The model under review builds one solid part; all positions refer to its coordinate system, in mm. A direction names the side the tool comes from. Coordinates: 2 decimals unless noted, no trailing zeros. Write each loop counter-clockwise with the first axis right and the second up, starting at its lowest first coordinate (ties: lowest second). Pieces come first, ordered by that corner, then holes. Notation, with made-up numbers: (79.5, 34) - (86.5, 34) arc R12 ccw to (86.5, 42) - close; hole circle Ø7 at (82.25, 85.25). An arc over 180 degrees is marked (long way). Return JSON: item names as keys, results as strings. Group by question number.
(1) For pin 1 Ø12 at (y, z) = (-9, 12) entering from +X; pin 2 Ø3 at (x, z) = (-2.5, 12) entering from -Y; pin 3 Ø1.5 at (y, z) = (-12.5, 15.5) entering from +X, all flat-tipped, find the tip position at first contact; note any pin that passes through.
(2) To check wall thickness, follow L1, parallel to Z at x = -10.5, y = -15; L2, parallel to X at y = 15.25, z = 9.5; L3, parallel to Y at x = 15.25, z = -1.5. State the ranges of each line that lie inside material, in increasing order. Write a range as from..to.
(3) We need section B-B on x = 15.25. Give the number of separate pieces and of enclosed holes in the cut face, then the cut area to 3 significant figures.
(4) We need section C-C on y = -7.5. State the section outline as (x, z) points.
(5) Draft analysis for pull direction Y (two halves, no side actions). For faces 1 (the face through (-18, 0, 10)), 2 (the face through (0, 0, 2)), 3 (the face through (0, 18, 10)), state which applies: released by +Y, released by -Y, zero draft, split by the parting line, or undercut.
(6) We need section A-A on z = 4.25. State the section outline as (x, y) points, then the cut area to 3 significant figures.
(7) We need section D-D on x = -6.5. State the section outline as (y, z) points, then the cut area to 3 significant figures.
(8) Tool access review of faces 4 (the face through (-17.551, 17.015, -2.465)), 5 (the face through (17.5, 17.5, 0)), 6 (the face through (-17.551, -17.015, 5.451)): name each direction out of +Z, -Z, +X, -X, +Y, -Y from which nothing blocks a thin tool from reaching the whole face with its end or side.
```python
from build123d import *

# Parameters (mm, degrees)
SKETCH_W      = 36
SKETCH_H      = 36
SKETCH_R      = 1.5
PAD_DEPTH     = 2
SKETCH001_R   = 2.9
SKETCH001_R_2 = 1.5
PAD001_DEPTH  = 7
SKETCH002_W   = 36
SKETCH002_H   = 36
SKETCH002_R   = 1.5
PAD002_DEPTH  = 2
SKETCH003_R   = 2.9
SKETCH003_R_2 = 1.5
PAD003_DEPTH  = 5
SKETCH004_W   = 18
SKETCH004_H   = 36
PAD004_DEPTH  = 2
SKETCH005_R   = 2.9
SKETCH005_R_2 = 1.5
PAD005_DEPTH  = 5


with BuildPart() as part:
    # Sketch → Pad (new body)
    with BuildSketch(Plane.XY):
        Rectangle(SKETCH_W, SKETCH_H)
        with Locations((-15.25, -15.25)):
            Circle(SKETCH_R, mode=Mode.SUBTRACT)
        with Locations((15.25, -15.25)):
            Circle(SKETCH_R, mode=Mode.SUBTRACT)
        with Locations((-15.25, 15.25)):
            Circle(SKETCH_R, mode=Mode.SUBTRACT)
        with Locations((15.25, 15.25)):
            Circle(SKETCH_R, mode=Mode.SUBTRACT)
    extrude(amount=PAD_DEPTH)

    # Sketch001 (on Face10 of Pad) → Pad001 (join)
    with BuildSketch(Plane.XY.offset(2)):
        with Locations((-15.25, 15.25)):
            Circle(SKETCH001_R)
        with Locations((-15.25, 15.25)):
            Circle(SKETCH001_R_2, mode=Mode.SUBTRACT)
        with Locations((-15.25, -15.25)):
            Circle(SKETCH001_R)
        with Locations((-15.25, -15.25)):
            Circle(SKETCH001_R_2, mode=Mode.SUBTRACT)
        with Locations((15.25, -15.25)):
            Circle(SKETCH001_R)
        with Locations((15.25, -15.25)):
            Circle(SKETCH001_R_2, mode=Mode.SUBTRACT)
        with Locations((15.25, 15.25)):
            Circle(SKETCH001_R)
        with Locations((15.25, 15.25)):
            Circle(SKETCH001_R_2, mode=Mode.SUBTRACT)
    extrude(amount=PAD001_DEPTH)

    # Sketch002 (on Face31 of Pad001) → Pad002 (join)
    with BuildSketch(Plane.XY.offset(9)):
        Rectangle(SKETCH002_W, SKETCH002_H)
        with Locations((-15.25, 15.25)):
            Circle(SKETCH002_R, mode=Mode.SUBTRACT)
        with Locations((15.25, 15.25)):
            Circle(SKETCH002_R, mode=Mode.SUBTRACT)
        with Locations((15.25, -15.25)):
            Circle(SKETCH002_R, mode=Mode.SUBTRACT)
        with Locations((-15.25, -15.25)):
            Circle(SKETCH002_R, mode=Mode.SUBTRACT)
    extrude(amount=PAD002_DEPTH)

    # Sketch003 (on Face52 of Pad002) → Pad003 (join)
    with BuildSketch(Plane.XY.offset(11)):
        with Locations((-15.25, 15.25)):
            Circle(SKETCH003_R)
        with Locations((-15.25, 15.25)):
            Circle(SKETCH003_R_2, mode=Mode.SUBTRACT)
        with Locations((-15.25, -15.25)):
            Circle(SKETCH003_R)
        with Locations((-15.25, -15.25)):
            Circle(SKETCH003_R_2, mode=Mode.SUBTRACT)
    extrude(amount=PAD003_DEPTH)

    # Sketch004 (on Face63 of Pad003) → Pad004 (join)
    with BuildSketch(Plane.XY.offset(16)):
        with Locations((-9, 0)):
            Rectangle(SKETCH004_W, SKETCH004_H)
    extrude(amount=PAD004_DEPTH)

    # Sketch005 (on Face4 of Pad004) → Pad005 (join)
    with BuildSketch(Plane(origin=(0, 0, 0), x_dir=(1, 0, 0), z_dir=(0, 0, -1))):
        with Locations((-15.25, 15.25)):
            Circle(SKETCH005_R)
        with Locations((-15.25, 15.25)):
            Circle(SKETCH005_R_2, mode=Mode.SUBTRACT)
        with Locations((-15.25, -15.25)):
            Circle(SKETCH005_R)
        with Locations((-15.25, -15.25)):
            Circle(SKETCH005_R_2, mode=Mode.SUBTRACT)
        with Locations((15.25, -15.25)):
            Circle(SKETCH005_R)
        with Locations((15.25, -15.25)):
            Circle(SKETCH005_R_2, mode=Mode.SUBTRACT)
        with Locations((15.25, 15.25)):
            Circle(SKETCH005_R)
        with Locations((15.25, 15.25)):
            Circle(SKETCH005_R_2, mode=Mode.SUBTRACT)
    extrude(amount=PAD005_DEPTH)


solid = part.part
```
Ans:
{
 "1": {"pin 1": "x = 18", "pin 2": "y = -18", "pin 3": "x = 0"},
 "2": {"L1": "0..2, 9..11, 16..18", "L2": "-18..-16.75, -13.75..13.75, 16.75..18", "L3": "-18.15..-16.75, -13.75..-12.35, 12.35..13.75, 16.75..18.15"},
 "3": {"separate pieces": "3", "enclosed holes": "1", "area": "187 mm²"},
 "4": {"outline": "(-18, 0) - (18, 0) - (18, 2) - (-18, 2) - close; (-18, 9) - (18, 9) - (18, 11) - (-18, 11) - close; (-18, 16) - (0, 16) - (0, 18) - (-18, 18) - close"},
 "5": {"face 1": "zero draft", "face 2": "undercut", "face 3": "released by +Y"},
 "6": {"outline": "circle Ø5.8 at (-15.25, -15.25); circle Ø5.8 at (-15.25, 15.25); circle Ø5.8 at (15.25, -15.25); circle Ø5.8 at (15.25, 15.25); hole circle Ø3 at (-15.25, -15.25); hole circle Ø3 at (-15.25, 15.25); hole circle Ø3 at (15.25, -15.25); hole circle Ø3 at (15.25, 15.25)", "area": "77.4 mm²"},
 "7": {"outline": "(-18, 0) - (18, 0) - (18, 2) - (-18, 2) - close; (-18, 9) - (18, 9) - (18, 11) - (-18, 11) - close; (-18, 16) - (18, 16) - (18, 18) - (-18, 18) - close", "area": "216 mm²"},
 "8": {"face 4": "-Z", "face 5": "-Z, +X, +Y", "face 6": "none"}
}
